from build123d import *

# Parameters (mm, degrees)
F0_W      = 400
F0_H      = 250
F1_DEPTH  = 127
F2_R      = 50
F3_DEPTH  = 150
F5_D      = 11
F7_D      = 14
F8_DEPTH  = 254
F9_R      = 5.08
F11_DEPTH = 250.001
F12_W     = 127
F12_H     = 76.4771783382
F13_DEPTH = 25.4
F14_W     = 30
F14_H     = 30
F14_R     = 30
F15_DEPTH = 277.001


with BuildPart() as f1:
    # F0 (on Top) → F1 (new body)
    with BuildSketch(Plane.XY):
        with Locations((-200, -125)):
            Rectangle(F0_W, F0_H)
    extrude(amount=F1_DEPTH)

    # F2 (on face) → F3 (join)
    with BuildSketch(Plane(origin=(0, 0, 0), x_dir=(1, 0, 0), z_dir=(0, 0, -1))):
        with Locations((-300, 100)):
            Circle(F2_R)
    extrude(amount=F3_DEPTH)

    # F5 (through all)
    with Locations(Plane(origin=(0, 0, 0), x_dir=(1, 0, 0), z_dir=(0, 0, -1))):
        with Locations((-400, 220), (-100, 220)):
            Hole(F5_D / 2)

    # F7 (through all)
    with Locations(Plane.XZ.offset(250)):
        with Locations((-381, 76.2), (-254, 75.1730280948)):
            Hole(F7_D / 2)

    # F8 (add): a face of the model
    f8_faces = [f1.faces().sort_by_distance(p)[0] for p in [
        (0, -125, 63.5),
    ]]
    extrude(f8_faces, amount=F8_DEPTH)

    # F9
    f9_edges = [f1.edges().sort_by_distance(p)[0] for p in [
        (254, -250, 63.5),
        (254, 0, 63.5),
        (254, -125, 0),
        (254, -125, 127),
        (-73, -250, 127),
    ]]
    fillet(f9_edges, radius=F9_R)

    # F10 (on face) → F11 (cut, through all)
    with BuildSketch(Plane(origin=(0, 0, 0), x_dir=(-1, 0, 0), z_dir=(0, 1, 0))):
        Polygon((-50.8, 127), (-165.6154772818, 127), (-165.6154772818, 50.8), (-101.6, 50.8), (-101.6, 76.2), (-50.8, 76.2), align=None)
    extrude(amount=-F11_DEPTH, mode=Mode.SUBTRACT)

    # F12 (on face) → F13 (join)
    with BuildSketch(Plane.XY.offset(127)):
        with Locations((55.3710968234, -193.1489035487)):
            Rectangle(F12_W, F12_H)
    extrude(amount=F13_DEPTH)

    # F14 (on face) → F15 (cut, through all)
    with BuildSketch(Plane.XY.offset(127)):
        with Locations((-185, -120)):
            Rectangle(F14_W, F14_H)
        with Locations((-185, -180)):
            Rectangle(F14_W, F14_H)
        with Locations((-280, -150)):
            Circle(F14_R)
    extrude(amount=-F15_DEPTH, mode=Mode.SUBTRACT)


solid = f1.part
Design review of the part built by this model. Coordinates are the model's own, in mm. A direction names the side the tool comes from. Coordinates: 2 decimals unless noted, no trailing zeros. Loops run counter-clockwise (first coordinate to the right, second up) from the corner with the lowest first, then second, coordinate; pieces in that order, holes last.
Item 1: Add section B-B (x = -381). Write out the cut boundary in (y, z), and give its area (3 significant figures).
Completed:
outline: (-250, 0) - (0, 0) - (0, 69.2) - (-250, 69.2) - close; (-250, 83.2) - (0, 83.2) - (0, 127) - (-244.92, 127) arc R5.08 ccw to (-250, 121.92) - close
area: 28,200 mm2
Item 2: Add section D-D (x = -187). Write out the cut boundary in (y, z), and give its area (3 significant figures).
Completed:
outline: (-250, 0) - (-195, 0) - (-195, 127) - (-244.92, 127) arc R5.08 ccw to (-250, 121.92) - close; (-165, 0) - (-135, 0) - (-135, 127) - (-165, 127) - close; (-105, 0) - (0, 0) - (0, 127) - (-105, 127) - close
area: 24,100 mm2
Item 3: Clearance check with flat-ended pins moving along their axes: pin 1 (12.5 mm diameter, centred on y = -182.5, z = 145, fed in from +X); pin 2 (8.5 mm diameter, centred on x = -254, z = 75.17, fed in from +Y); pin 3 (6 mm diameter, centred on x = -54.5, y = -174, fed in from +Z); pin 4 (15 mm diameter, centred on x = 77.5, y = -84, fed in from +Z). State where each tip first meets the part, or that it passes through.
Completed:
pin 1: stops at x = 118.87
pin 2: passes through
pin 3: stops at z = 127
pin 4: stops at z = 76.2
Item 4: For faces 4 (the flat face through (77, -123, 76.2)), 5 (the flat face through (165.615, -123, 89)), 6 (the flat face through (-8.129, -194, 140)), 7 (the flat face through (118.871, -194, 140)), list the 3-axis set-ups (+Z, -Z, +X, -X, +Y, -Y) from which the entire face can be reached by the end or side of a thin tool; tool diameter is ignored.
Completed:
face 4: +Y, -Y
face 5: +Z, +Y, -Y
face 6: +Z, -X, +Y, -Y
face 7: +Z, +X, +Y, -Y
Item 5: Add section A-A (z = 61). Write out the cut boundary in (x, y), and give its area (3 significant figures).
Completed:
outline: (-400, -250) - (101.6, -250) - (101.6, 0) - (-400, 0) - (-400, -214.5) arc R5.5 cw to (-400, -225.5) - close; (165.62, -250) - (248.92, -250) arc R5.08 ccw to (254, -244.92) - (254, -5.08) arc R5.08 ccw to (248.92, 0) - (165.62, 0) - close; hole circle Ø60 at (-280, -150); hole (-200, -195) - (-170, -195) - (-170, -165) - (-200, -165) - close; hole (-200, -135) - (-170, -135) - (-170, -105) - (-200, -105) - close; hole circle Ø11 at (-100, -220)
area: 143,000 mm2
Item 6: Add section C-C (z = 109). Write out the cut boundary in (x, y), and give its area (3 significant figures).
Completed:
outline: (-400, -250) - (50.8, -250) - (50.8, 0) - (-400, 0) - (-400, -214.5) arc R5.5 cw to (-400, -225.5) - close; (165.62, -250) - (248.92, -250) arc R5.08 ccw to (254, -244.92) - (254, -5.08) arc R5.08 ccw to (248.92, 0) - (165.62, 0) - close; hole circle Ø60 at (-280, -150); hole (-200, -195) - (-170, -195) - (-170, -165) - (-200, -165) - close; hole (-200, -135) - (-170, -135) - (-170, -105) - (-200, -105) - close; hole circle Ø11 at (-100, -220)
area: 130,000 mm2
Item 7: Draft analysis for pull direction Y (two halves, no side actions). For faces 1 (the flat face through (54, -231.387, 140)), 2 (the flat face through (-400, -109, 63)), 3 (the flat face through (-170, -120, 64)), state which applies: pulls with the +Y half, pulls with the -Y half, needs draft (parallel to the pull), parting line crosses it, or undercut.
Completed:
face 1: pulls with the -Y half
face 2: needs draft
face 3: undercut
Item 8: Wall thickness on L1, parallel to X at y = -220, z = 97.5; L2, parallel to X at y = -150, z = 53.5; L3, parallel to Z at x = -381, y = -146.5: over which ranges is each line inside the solid? List them lowest first.
Completed:
L1: x = -394.5 to -105.5, -94.5 to 50.8, 165.62 to 254
L2: x = -400 to -310, -250 to 101.6, 165.62 to 254
L3: z = 0 to 69.2, 83.2 to 127
